Can you work these out from the model? Positions are in its coordinate system, mm. Face numbers are marked on the shaded views. A direction names the side the tool comes from. Coordinates: 2 decimals unless noted, no trailing zeros. Write each loop counter-clockwise with the first axis right and the second up, starting at its lowest first coordinate (ties: lowest second). Pieces come first, ordered by that corner, then holes. Notation, with made-up numbers: M 88.5,71.5 L 123.5,71.5 A9 ccw 123.5,88.5 Z; hole C 50,85.5 d4. An arc over 180 degrees is marked long. Use one line per item in the form item = value. Start each with the question number.
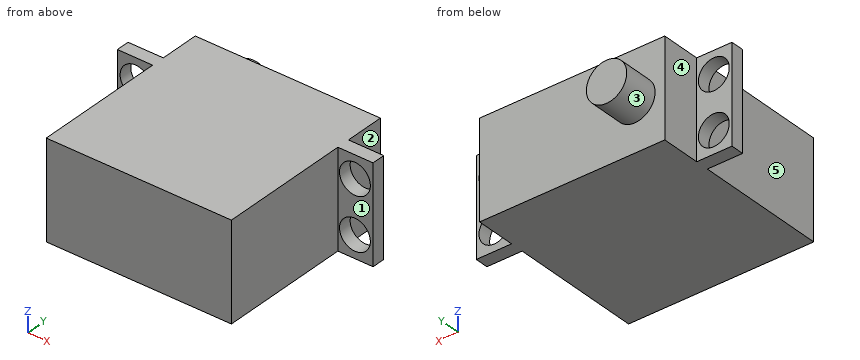
```python
from build123d import *

# Parameters (mm, degrees)
SKETCH_1_W          = 42
SKETCH_1_H          = 22
EXTRUDE_1_DEPTH     = 42
SKETCH_2_W          = 8
SKETCH_2_H          = 22
EXTRUDE_2_DEPTH     = 3
SKETCH_3_R          = 3.5
CUT_EXTRUDE_1_DEPTH = 3
SKETCH_4_R          = 4.581673227
EXTRUDE_3_DEPTH     = 8


with BuildPart() as part:
    # 草图1 → 凸台-拉伸1 (new body)
    with BuildSketch(Plane(origin=(0, 0, 0), x_dir=(1, 0, 0), z_dir=(0, 1, 0))):
        Rectangle(SKETCH_1_W, SKETCH_1_H)
    extrude(amount=EXTRUDE_1_DEPTH)

    # 草图2 → 凸台-拉伸2 (add)
    with BuildSketch(Plane(origin=(0, 30, 0), x_dir=(1, 0, 0), z_dir=(0, 1, 0))):
        with Locations((-25, 0)):
            Rectangle(SKETCH_2_W, SKETCH_2_H)
        with Locations((25, 0)):
            Rectangle(SKETCH_2_W, SKETCH_2_H)
    extrude(amount=EXTRUDE_2_DEPTH)

    # 草图3 → 切除-拉伸1 (cut)
    with BuildSketch(Plane(origin=(0, 33, 0), x_dir=(1, 0, 0), z_dir=(0, 1, 0))):
        with Locations(Location((-24.879659127, -5.919206434, 0), (0, 0, 270))):
            Circle(SKETCH_3_R)
        with Locations(Location((-24.879659127, 5.919206434, 0), (0, 0, 270))):
            Circle(SKETCH_3_R)
        with Locations(Location((24.879659127, 5.919206434, 0), (0, 0, 270))):
            Circle(SKETCH_3_R)
        with Locations(Location((24.879659127, -5.919206434, 0), (0, 0, 270))):
            Circle(SKETCH_3_R)
    extrude(amount=-CUT_EXTRUDE_1_DEPTH, mode=Mode.SUBTRACT)

    # 草图4 → 凸台-拉伸3 (add)
    with BuildSketch(Plane(origin=(0, 42, 0), x_dir=(1, 0, 0), z_dir=(0, 1, 0))):
        with Locations(Location((-14.223956567, 0, 0), (0, 0, 270))):
            Circle(SKETCH_4_R)
    extrude(amount=EXTRUDE_3_DEPTH)


solid = part.part
```
1) Suppose I cut it at A-A on z = -3.25. Please give me the cut outline in (x, y).
2) Suppose I cut it at C-C on x = -5. Please give me the cut outline in (y, z), and give its area (3 significant figures).
3) Which directions (+Z, -Z, +X, -X, +Y, -Y) give clear straight access to the entire face, cutting with the end or side of a thin tool? Please do the marked faces 1, 2, 3, 4 and 5.
4) Suppose I cut it at D-D on z = 7.25. Please give me the cut outline in (x, y).
5) Please list where these lines run through material, in increasing order: line 1 (X direction, y = 37, z = -3.5); line 2 (Y direction, x = -5, z = -1.5); line 3 (Y direction, x = 25, z = -0.5).
6) Suppose I cut it at B-B on z = 0. Please give me the cut outline in (x, y).
7) Will these pins go through, and if not, where does the flat tip stop? pin 1 Ø1 at (x, z) = (-14, 8.5) entering from +Y; pin 2 Ø4 at (y, z) = (42.5, 0) entering from -X; pin 3 Ø4 at (x, z) = (-25.5, -4.5) entering from -Y.
Computed values:
q1.outline = M -29,30 L -27.14,30 L -27.14,33 L -29,33 Z; M -22.62,30 L -21,30 L -21,0 L 21,0 L 21,30 L 22.62,30 L 22.62,33 L 21,33 L 21,42 L -10.99,42 L -10.99,50 L -17.45,50 L -17.45,42 L -21,42 L -21,33 L -22.62,33 Z; M 27.14,30 L 29,30 L 29,33 L 27.14,33 Z
q2.outline = M 0,-11 L 42,-11 L 42,11 L 0,11 Z
q2.area = 924 mm²
q3.face_1 = +Z, -Z, +X, -Y
q3.face_2 = +Z, -Z, +X, +Y
q3.face_3 = +Y
q3.face_4 = +Z, -Z, -X, +Y
q3.face_5 = +Z, -Z, -X, -Y
q4.outline = M -29,30 L -28.12,30 L -28.12,33 L -29,33 Z; M -21.64,30 L -21,30 L -21,0 L 21,0 L 21,30 L 21.64,30 L 21.64,33 L 21,33 L 21,42 L -21,42 L -21,33 L -21.64,33 Z; M 28.12,30 L 29,30 L 29,33 L 28.12,33 Z
q5.line_1 = -21 to 21
q5.line_2 = 0 to 42
q5.line_3 = 30 to 33
q6.outline = M -29,30 L -21,30 L -21,0 L 21,0 L 21,30 L 29,30 L 29,33 L 21,33 L 21,42 L -9.64,42 L -9.64,50 L -18.81,50 L -18.81,42 L -21,42 L -21,33 L -29,33 Z
q7.pin_1 = 42
q7.pin_2 = -21
q7.pin_3 = 30
